Source: three-view drawing plus pictorial views. Frame: mm from the lowest corner of the part. A direction names the side the tool comes from. Give positions to 0.01 mm unless a question says otherwise; leave off trailing zeros. Write each loop counter-clockwise with the first axis right and the second up, starting at its lowest first coordinate (ties: lowest second). Pieces come first, ordered by that corner, then holes. Notation, with made-up numbers: (22.25, -5.5) -> (57.25, -5.5) arc R27 cw to (57.25, 31.5) -> close; hole circle Ø5 at (75, -33.75). An arc over 180 degrees is marked (long way). Answer in a Markdown table with one row per item. Add a question column.
Item 1: Section query B-B on x = 17.5. Output: boundary loops of the cut face in (y, z), plus the area to 3 significant figures.
Item 2: Section query A-A on y = 11. Output: boundary loops of the cut face in (x, z), plus the area to 3 significant figures.
Item 3: Section query C-C on z = 4.75. Output: boundary loops of the cut face in (x, y).
Item 4: Material intervals for probe 1 along Y at (x, z) = (11, 6); probe 2 along Y at (x, z) = (5.25, 4.05); probe 3 along Z at (x, y) = (3.5, 11.25), sorted ascending. Write a range as from..to.
Item 5: Access query for the marked faces 5, 6 and 7. Directions: +Z, -Z, +X, -X, +Y, -Y. A direction counts if a zero-diameter tool reaches every point of the face in a straight line with its end or side. Return the directions, or none.
Item 6: First-contact query: P1, Ø4, axis at x = 16.75, y = 5.25, coming from the -Z side; P2, Ø4, axis at x = 10, z = 13, coming from the +Y side; P3, Ø1, axis at y = 14.5, z = 11.5, coming from the +X side. Flat tips, straight axial feed; report the tip coordinate or a pass-through.
Item 7: Draft query along X for the marked faces 1, 2, 3 and 4. Return one class per face: +X half, -X half, draft (parallel to the pull), parting line (faces both ways), or undercut.
Item 8: Section query D-D on x = 11.75. Output: boundary loops of the cut face in (y, z), plus the area to 3 significant figures.
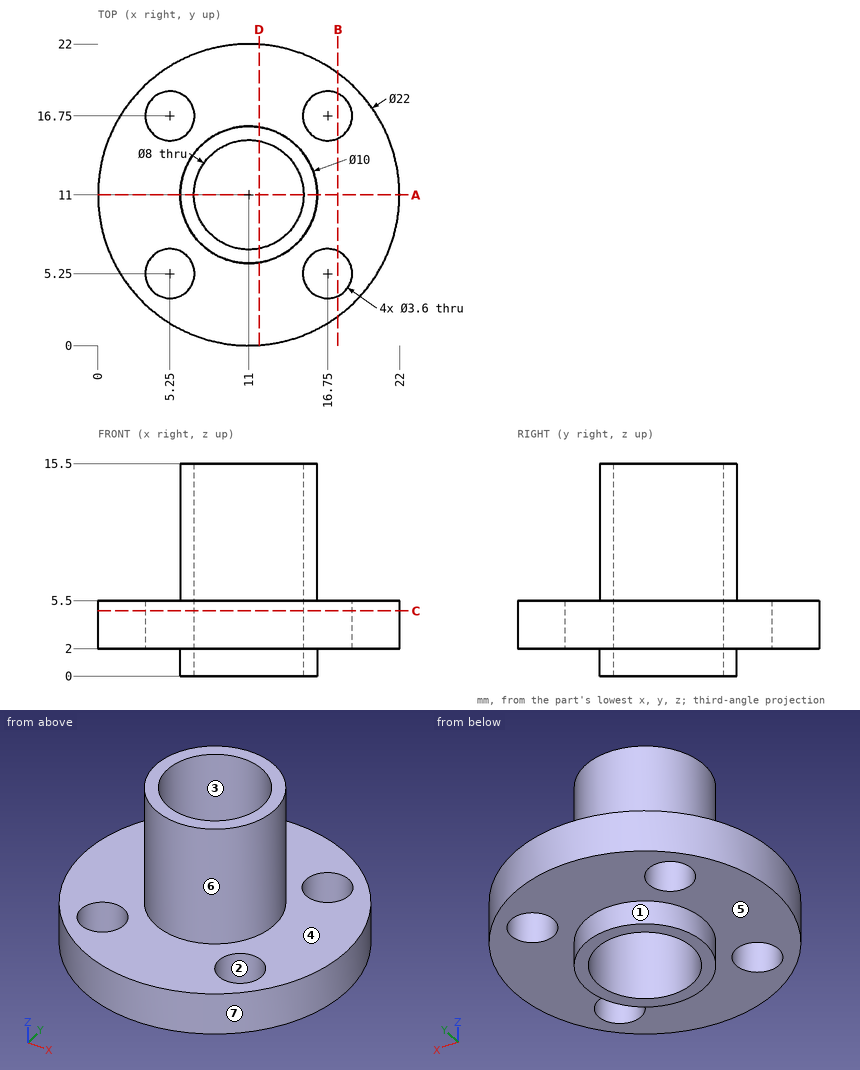
Findings below:
| question | item | result |
|---|---|---|
| 1 | outline | (2.13, 2) -> (3.61, 2) -> (3.61, 5.5) -> (2.13, 5.5) -> close; (6.89, 2) -> (15.11, 2) -> (15.11, 5.5) -> (6.89, 5.5) -> close; (18.39, 2) -> (19.87, 2) -> (19.87, 5.5) -> (18.39, 5.5) -> close |
| 1 | area | 39.2 mm^2 |
| 2 | outline | (0, 2) -> (6, 2) -> (6, 0) -> (7, 0) -> (7, 15.5) -> (6, 15.5) -> (6, 5.5) -> (0, 5.5) -> close; (15, 0) -> (16, 0) -> (16, 2) -> (22, 2) -> (22, 5.5) -> (16, 5.5) -> (16, 15.5) -> (15, 15.5) -> close |
| 2 | area | 73.0 mm^2 |
| 3 | outline | circle Ø22 at (11, 11); hole circle Ø3.6 at (5.25, 5.25); hole circle Ø3.6 at (5.25, 16.75); hole circle Ø8 at (11, 11); hole circle Ø3.6 at (16.75, 5.25); hole circle Ø3.6 at (16.75, 16.75) |
| 4 | probe 1 | y = 6..7, 15..16 |
| 4 | probe 2 | y = 1.62..3.45, 7.05..14.95, 18.55..20.38 |
| 4 | probe 3 | z = 2..5.5 |
| 5 | face 5 | -Z |
| 5 | face 6 | +Z |
| 5 | face 7 | +Z, -Z |
| 6 | P1 | stops at z = 2 |
| 6 | P2 | stops at y = 16 |
| 6 | P3 | stops at x = 15 |
| 7 | face 1 | parting line |
| 7 | face 2 | undercut |
| 7 | face 3 | undercut |
| 7 | face 4 | draft |
| 8 | outline | (0.03, 2) -> (6.06, 2) -> (6.06, 0) -> (7.07, 0) -> (7.07, 15.5) -> (6.06, 15.5) -> (6.06, 5.5) -> (0.03, 5.5) -> close; (14.93, 0) -> (15.94, 0) -> (15.94, 2) -> (21.97, 2) -> (21.97, 5.5) -> (15.94, 5.5) -> (15.94, 15.5) -> (14.93, 15.5) -> close |
| 8 | area | 73.7 mm^2 |
